For this review, take the finished solid that the model builds, in its own axes (mm). Round coordinates to 2 decimals unless told otherwise and drop trailing zeros. Order: outer loops, then holes, each group sorted by start corner. A loop starts at its lowest first (then second) coordinate and runs counter-clockwise, first axis right, second up. Notation, with made-up numbers: (7, -4) - (51, -4) arc R27 cw to (51, 12) - close; hole circle Ø2 at (-31.75, 60). An arc over 180 degrees is marked (long way). One line per question, with ' | ' between items.
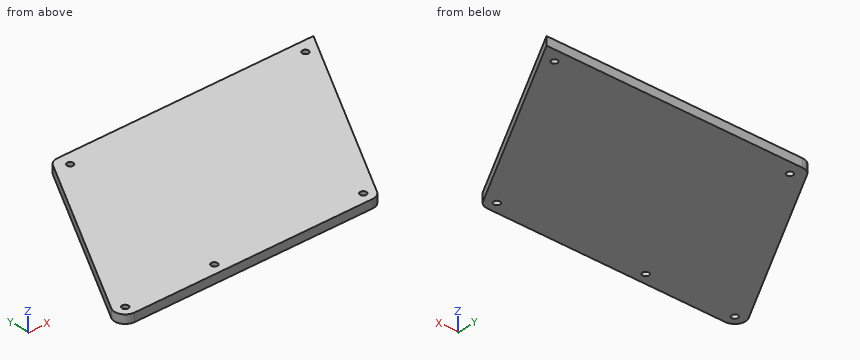
```python
from build123d import *

# Parameters (mm, degrees)
BOSS_EXTRU_1_DEPTH      = 8
ESQUISSE2_R             = 3
ENL_V_MAT_EXTRU_1_DEPTH = 1597.033446326


with BuildPart() as part:
    # Esquisse1 → Boss.-Extru.1 (new body)
    with BuildSketch(Plane.XY):
        with BuildLine():
            Line((5.773502692, 0), (250, 0))
            Line((250, 0), (143.1902002, -185))
            ThreePointArc((143.1902002, -185), (139.529946162, -188.660254038), (134.529946162, -190))
            Line((134.529946162, -190), (-92.37604307, -190))
            ThreePointArc((-92.37604307, -190), (-101.036297108, -185), (-101.036297108, -175))
            Line((-101.036297108, -175), (-2.886751346, -5))
            ThreePointArc((-2.886751346, -5), (0.773502692, -1.339745962), (5.773502692, 0))
        make_face()
    extrude(amount=BOSS_EXTRU_1_DEPTH)

    # Esquisse2 → Enlèv. mat.-Extru.1 (cut, through all)
    with BuildSketch(Plane(origin=(-1216.410161514, -630, 8), x_dir=(1, 0, 0), z_dir=(0, 0, 1))):
        with Locations((1124.034118443, 450)):
            Circle(ESQUISSE2_R)
        with Locations((1209.034118443, 450)):
            Circle(ESQUISSE2_R)
        with Locations((1223.481958283, 618)):
            Circle(ESQUISSE2_R)
        with Locations((1447.9349529, 618)):
            Circle(ESQUISSE2_R)
        with Locations((1350.940107676, 450)):
            Circle(ESQUISSE2_R)
    extrude(amount=-ENL_V_MAT_EXTRU_1_DEPTH, mode=Mode.SUBTRACT)


solid = part.part
```
(1) For probe 1 along Y at (x, z) = (7, 6.25); probe 2 along X at (y, z) = (-180, 4.5); probe 3 along X at (y, z) = (-29, 0.75), list the stretches that pass through material, from the lowest coordinate up. Write a range as [from, to].
Output values:
probe 1: [-190, -15], [-9, 0] | probe 2: [-102.38, -95.38], [-89.38, -10.38], [-4.38, 131.53], [137.53, 146.08] | probe 3: [-16.74, 233.26]
(2) We need section C-C on y = -139.5. State the section outline as (x, z) points.
Output values:
outline: (-80.54, 0) - (169.46, 0) - (169.46, 8) - (-80.54, 8) - close
(3) We need section A-A on z = 4. State the section outline as (x, y) points, plus the area to 3 significant figures.
Output values:
outline: (-101.04, -175) arc R10 ccw to (-92.38, -190) - (134.53, -190) arc R10 ccw to (143.19, -185) - (250, 0) - (5.77, 0) arc R10 ccw to (-2.89, -5) - close; hole circle Ø6 at (-92.38, -180); hole circle Ø6 at (-7.38, -180); hole circle Ø6 at (7.07, -12); hole circle Ø6 at (134.53, -180); hole circle Ø6 at (231.52, -12) | area: 47,300 mm^2
(4) We need section B-B on x = 148.5. State the section outline as (y, z) points, plus the area to 3 significant figures.
Output values:
outline: (-175.8, 0) - (0, 0) - (0, 8) - (-175.8, 8) - close | area: 1,410 mm^2
(5) Insertion check: pin 1 (3 mm diameter, centred on y = -140, z = 3.5, fed in from +X); pin 2 (9.5 mm diameter, centred on x = 7.07, y = -12, fed in from +Z); pin 3 (1.5 mm diameter, centred on y = -122, z = 4, fed in from +X). Each pin has a flat end and moves straight along its axis. Give the tip position at first contact, or say it passes through.
Output values:
pin 1: x = 170.04 | pin 2: z = 8 | pin 3: x = 180
